Study the drawing (mm; zero at the part's minimum x, y, z) and answer. A direction names the side the tool comes from. Round coordinates to 2 decimals unless told otherwise and drop trailing zeros. Write each loop counter-clockwise with the first axis right and the second up, starting at its lowest first coordinate (ties: lowest second). Pieces come first, ordered by that corner, then holes.
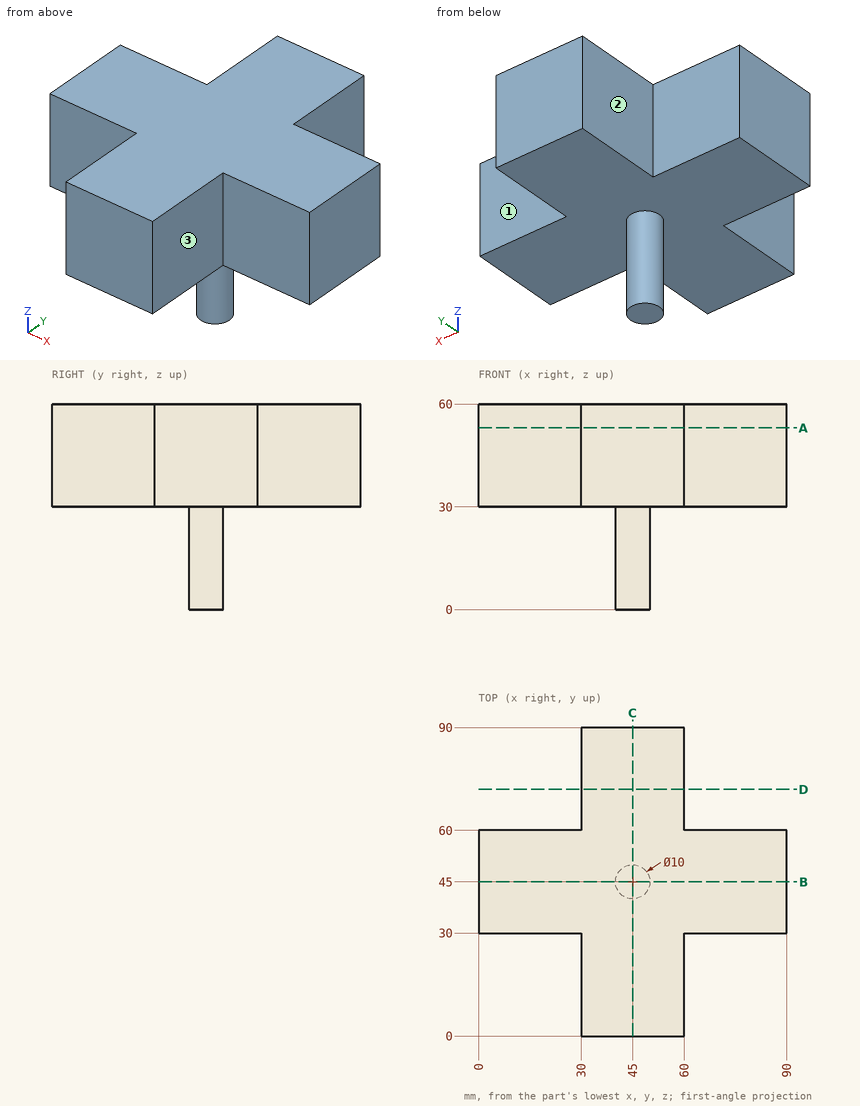
1. A tool of negligible diameter and unlimited length cuts with its end or side. For the marked faces 1, 2 and 3, from which of +Z, -Z, +X, -X, +Y, -Y can it reach the whole face along a straight path? Write none if from no direction.
Geometry says:
face 1: +Z, -Z, +X, +Y
face 2: +Z, -Z, -X, +Y
face 3: +Z, -Z, +X, -Y
2. Section A-A on z = 53 is taken. Determine the outline of the cut face in (x, y), plus the area to 3 significant figures.
Geometry says:
outline: (0, 30) - (30, 30) - (30, 0) - (60, 0) - (60, 30) - (90, 30) - (90, 60) - (60, 60) - (60, 90) - (30, 90) - (30, 60) - (0, 60) - close
area: 4,500 mm2
3. Section B-B on y = 45 is taken. Determine the outline of the cut face in (x, z).
Geometry says:
outline: (0, 30) - (40, 30) - (40, 0) - (50, 0) - (50, 30) - (90, 30) - (90, 60) - (0, 60) - close
4. A straight line is drawn through the part: line 1 along Y through (x, z) = (64, 49.5). Find the intervals that lie inside material, in ascending order.
Geometry says:
line 1: y = 30 to 60
5. Given pin 1 (15 mm diameter, centred on x = 81.5, z = 46, fed in from -Y); pin 2 (15 mm diameter, centred on y = 9, z = 41, fed in from +X); pin 3 (2 mm diameter, centred on y = 39.5, z = 27.5, fed in from +X), each flat-ended and moving along its own axis, determine where each tip first touches the part or whether it passes through.
Geometry says:
pin 1: stops at y = 30
pin 2: stops at x = 60
pin 3: stops at x = 47.18
6. Section D-D on y = 72 is taken. Determine the outline of the cut face in (x, z), plus the area to 3 significant figures.
Geometry says:
outline: (30, 30) - (60, 30) - (60, 60) - (30, 60) - close
area: 900 mm2
